from build123d import *

# Parameters (mm, degrees)
SKETCH1_R           = 4.7
BOSS_EXTRUDE1_DEPTH = 20
SKETCH2_OUTSIDE_W   = 16.202
SKETCH2_OUTSIDE_H   = 16.202
SKETCH2_OUTSIDE_R   = 3.45
CUT_EXTRUDE1_DEPTH  = 5
SKETCH4_OUTSIDE_W   = 16.202
SKETCH4_OUTSIDE_H   = 16.202
SKETCH4_OUTSIDE_R   = 3.4
CUT_EXTRUDE2_DEPTH  = 12
SKETCH5_OUTSIDE_W   = 16.202
SKETCH5_OUTSIDE_H   = 16.202
SKETCH5_OUTSIDE_R   = 2.85
CUT_EXTRUDE3_DEPTH  = 3.3
SKETCH7_OUTSIDE_W   = 16.202
SKETCH7_OUTSIDE_H   = 16.202
SKETCH7_OUTSIDE_R   = 2.1
CUT_EXTRUDE4_DEPTH  = 2.5
CHAMFER1_SIZE       = 1
CHAMFER1_SIZE2      = 0.577350269


with BuildPart() as part:
    # Sketch1 → Boss-Extrude1 (new body)
    with BuildSketch(Plane(origin=(0, 0, 0), x_dir=(1, 0, 0), z_dir=(0, 1, 0))):
        with Locations(Location((0, 0, 0), (0, 0, 270))):  # turned: the seam where the file's is
            Circle(SKETCH1_R)
    extrude(amount=BOSS_EXTRUDE1_DEPTH)

    # Sketch2 outside → Cut-Extrude1 (cut)
    with BuildSketch(Plane.XZ):
        Rectangle(SKETCH2_OUTSIDE_W, SKETCH2_OUTSIDE_H)
        with Locations(Location((0, 0, 0), (0, 0, 270))):  # turned: the seam where the file's is
            Circle(SKETCH2_OUTSIDE_R, mode=Mode.SUBTRACT)
    extrude(amount=-CUT_EXTRUDE1_DEPTH, mode=Mode.SUBTRACT)

    # Sketch4 outside → Cut-Extrude2 (cut)
    with BuildSketch(Plane(origin=(0, 20, 0), x_dir=(1, 0, 0), z_dir=(0, 1, 0))):
        Rectangle(SKETCH4_OUTSIDE_W, SKETCH4_OUTSIDE_H)
        with Locations(Location((0, 0, 0), (0, 0, 270))):  # turned: the seam where the file's is
            Circle(SKETCH4_OUTSIDE_R, mode=Mode.SUBTRACT)
    extrude(amount=-CUT_EXTRUDE2_DEPTH, mode=Mode.SUBTRACT)

    # Sketch5 outside → Cut-Extrude3 (cut)
    with BuildSketch(Plane(origin=(0, 20, 0), x_dir=(1, 0, 0), z_dir=(0, 1, 0))):
        Rectangle(SKETCH5_OUTSIDE_W, SKETCH5_OUTSIDE_H)
        with Locations(Location((0, 0, 0), (0, 0, 270))):  # turned: the seam where the file's is
            Circle(SKETCH5_OUTSIDE_R, mode=Mode.SUBTRACT)
    extrude(amount=-CUT_EXTRUDE3_DEPTH, mode=Mode.SUBTRACT)

    # Sketch7 outside → Cut-Extrude4 (cut)
    with BuildSketch(Plane(origin=(0, 16.7, 0), x_dir=(1, 0, 0), z_dir=(0, 1, 0))):
        Rectangle(SKETCH7_OUTSIDE_W, SKETCH7_OUTSIDE_H)
        with Locations(Location((0, 0, 0), (0, 0, 270))):  # turned: the seam where the file's is
            Circle(SKETCH7_OUTSIDE_R, mode=Mode.SUBTRACT)
    extrude(amount=-CUT_EXTRUDE4_DEPTH, mode=Mode.SUBTRACT)

    # Chamfer1
    chamfer1_edges = [part.edges().sort_by_distance(p)[0] for p in [
        (0, 5, -4.7),
    ]]
    chamfer1_side = [part.faces().sort_by_distance(p)[0] for p in [
        (0, 6.5, -4.7),
    ]]
    chamfer(chamfer1_edges, length=CHAMFER1_SIZE, length2=CHAMFER1_SIZE2, reference=chamfer1_side[0])


solid = part.part
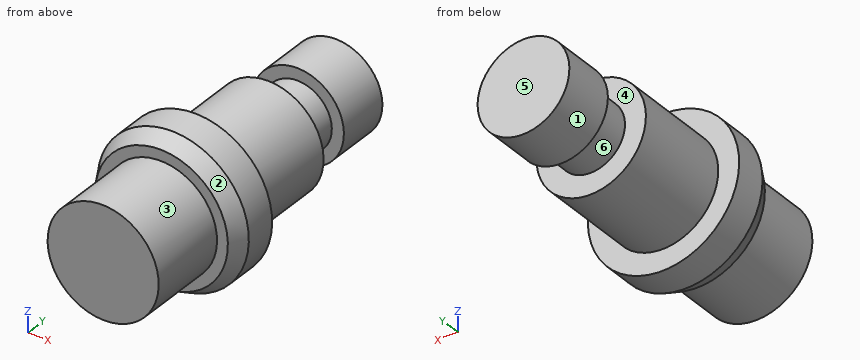
For this review, take the finished solid that the model builds, in its own axes (mm). Face numbers are marked on the shaded views. A direction names the side the tool comes from. Coordinates: 2 decimals unless noted, no trailing zeros. Loops run counter-clockwise (first coordinate to the right, second up) from the corner with the lowest first, then second, coordinate; pieces in that order, holes last. Notation, with made-up numbers: (5, 3) - (16, 3) arc R31 ccw to (16, 37) - close; hole circle Ø7 at (15, -14). An arc over 180 degrees is marked (long way). Use a Markdown table: item, result. Add a question column.
Item 1: We need section D-D (y = 10.75). Give the boundary of the cut face in (x, z), and give its area (3 significant figures).
Item 2: We need section C-C (y = 17.75). Give the boundary of the cut face in (x, z).
Item 3: Insertion check: pin 1 Ø4 at (y, z) = (16, 1) entering from -X; pin 2 Ø1 at (x, z) = (-2, 3) entering from +Y; pin 3 Ø3 at (x, y) = (-3, 7) entering from +Z. Each pin has a flat end and moves straight along its axis. Give the tip position at first contact, or say it passes through.
Item 4: For line 1 (Y direction, x = 1.75, z = -2.5); line 2 (Y direction, x = 2.25, z = -3.25); line 3 (X direction, y = 6.75, z = 2), list the stretches that pass through material, from the lowest coordinate up.
Item 5: Tool access review of the marked faces 1 and 2: name each direction out of +Z, -Z, +X, -X, +Y, -Y from which nothing blocks a thin tool from reaching the whole face with its end or side.
Item 6: We need section B-B (z = 0). Give the boundary of the cut face in (x, y), and give its area (3 significant figures).
Item 7: Mouldability with a two-part tool opening along Y and no side actions: class the marked faces 3, 4, 5 and 6 as pulls with the +Y half, pulls with the -Y half, needs draft (parallel to the pull), parting line crosses it, or undercut.
Item 8: We need section A-A (x = 0). Give the boundary of the cut face in (y, z).
Results list:
| question | item | result |
|---|---|---|
| 1 | outline | circle Ø6.8 at (0, 0) |
| 1 | area | 36.3 mm^2 |
| 2 | outline | circle Ø5.7 at (0, 0) |
| 3 | pin 1 | stops at x = -3.4 |
| 3 | pin 2 | stops at y = 14.2 |
| 3 | pin 3 | stops at z = 4.45 |
| 4 | line 1 | y = 0 to 14.2 |
| 4 | line 2 | y = 5 to 8 |
| 4 | line 3 | x = -4.25 to 4.25 |
| 5 | face 1 | +Y |
| 5 | face 2 | -Y |
| 6 | outline | (-4.7, 6) - (-4.12, 5) - (-3.45, 5) - (-3.45, 0) - (3.45, 0) - (3.45, 5) - (4.12, 5) - (4.7, 6) - (4.7, 8) - (3.4, 8) - (3.4, 14.2) - (2.1, 14.2) - (2.1, 16.7) - (2.85, 16.7) - (2.85, 20) - (-2.85, 20) - (-2.85, 16.7) - (-2.1, 16.7) - (-2.1, 14.2) - (-3.4, 14.2) - (-3.4, 8) - (-4.7, 8) - close |
| 6 | area | 134 mm^2 |
| 7 | face 3 | needs draft |
| 7 | face 4 | undercut |
| 7 | face 5 | pulls with the +Y half |
| 7 | face 6 | undercut |
| 8 | outline | (0, -3.45) - (5, -3.45) - (5, -4.12) - (6, -4.7) - (8, -4.7) - (8, -3.4) - (14.2, -3.4) - (14.2, -2.1) - (16.7, -2.1) - (16.7, -2.85) - (20, -2.85) - (20, 2.85) - (16.7, 2.85) - (16.7, 2.1) - (14.2, 2.1) - (14.2, 3.4) - (8, 3.4) - (8, 4.7) - (6, 4.7) - (5, 4.12) - (5, 3.45) - (0, 3.45) - close |
